Design review of the part built by this model. Coordinates are the model's own, in mm. Coordinates: 2 decimals unless noted, no trailing zeros. Loops run counter-clockwise (first coordinate to the right, second up) from the corner with the lowest first, then second, coordinate; pieces in that order, holes last. Notation, with made-up numbers: (52.5, 22.25) - (63.5, 22.25) arc R14 ccw to (63.5, 42.25) - close; hole circle Ø7 at (-18.75, 31). An arc over 180 degrees is marked (long way). Return JSON: item names as keys, results as strings. Group by question number.
from build123d import *

# Parameters (mm, degrees)
SKETCH_W     = 4.5
SKETCH_H     = 0.8
PAD_DEPTH    = 155
SKETCH002_W  = 8
SKETCH002_H  = 4
PAD001_DEPTH = 4


with BuildPart() as part:
    # Sketch → Pad (new body)
    with BuildSketch(Plane.XZ):
        Rectangle(SKETCH_W, SKETCH_H)
    extrude(amount=PAD_DEPTH)

    # Sketch002 (on Face4 of Pad) → Pad001 (join)
    with BuildSketch(Plane(origin=(0, 0, 0.4), x_dir=(-1, 0, 0), z_dir=(0, 0, 1))):
        with Locations((0, 153)):
            Rectangle(SKETCH002_W, SKETCH002_H)
        with Locations((0, 129.166667)):
            Rectangle(SKETCH002_W, SKETCH002_H)
        with Locations((0, 25.833333)):
            Rectangle(SKETCH002_W, SKETCH002_H)
        with Locations((0, 2)):
            Rectangle(SKETCH002_W, SKETCH002_H)
    extrude(amount=-PAD001_DEPTH)


solid = part.part
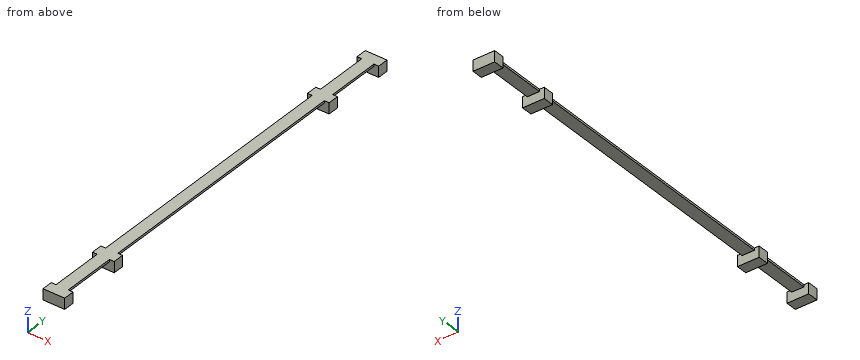
Item 1: Add section B-B (x = 1). State the section outline as (y, z) points.
Item 2: Add section A-A (z = -1.75). State the section outline as (x, y) points.
Item 3: Add section C-C (y = -104.5). State the section outline as (x, z) points, then the cut area to 3 significant figures.
Item 4: To check wall thickness, follow line 1 (Y direction, x = -1, z = -3.05); line 2 (Z direction, x = -1, y = -114); line 3 (X direction, y = -41, z = -0.15). State the ranges of each line that lie inside material, in increasing order. Write a range as from..to.
Item 5: For P1, Ø1.5, axis at y = -125, z = 0, coming from the +X side; P2, Ø0.6, axis at y = -143.5, z = 0, coming from the -X side; P3, Ø1.2, axis at x = 1.5, z = -2, coming from the +Y side; P4, Ø1.3, axis at x = -0.5, y = -10, coming from the -Z side, all flat-tipped, find the tip position at first contact; note any pin that passes through.
Answers below:
{
 "1": {"outline": "(-155, -3.6) - (-151, -3.6) - (-151, -0.4) - (-131.17, -0.4) - (-131.17, -3.6) - (-127.17, -3.6) - (-127.17, -0.4) - (-27.83, -0.4) - (-27.83, -3.6) - (-23.83, -3.6) - (-23.83, -0.4) - (-4, -0.4) - (-4, -3.6) - (0, -3.6) - (0, 0.4) - (-155, 0.4) - close"},
 "2": {"outline": "(-4, -155) - (4, -155) - (4, -151) - (-4, -151) - close; (-4, -131.17) - (4, -131.17) - (4, -127.17) - (-4, -127.17) - close; (-4, -27.83) - (4, -27.83) - (4, -23.83) - (-4, -23.83) - close; (-4, -4) - (4, -4) - (4, 0) - (-4, 0) - close"},
 "3": {"outline": "(-2.25, -0.4) - (2.25, -0.4) - (2.25, 0.4) - (-2.25, 0.4) - close", "area": "3.60 mm^2"},
 "4": {"line 1": "y = -155..-151, -131.17..-127.17, -27.83..-23.83, -4..0", "line 2": "z = -0.4..0.4", "line 3": "x = -2.25..2.25"},
 "5": {"P1": "stops at x = 2.25", "P2": "stops at x = -2.25", "P3": "stops at y = 0", "P4": "stops at z = -0.4"}
}
